Solid Edge part; units mm, degrees
sketch "Sketch1" plane through (0, 0, 2) normal (0, 0, 1) x (1, 0, 0)
  line L0 (49.4528, -16.8553) -> (36.691, -28.1957)
  arc A0 (31.6813, -30.1) -> (36.691, -28.1957) centre (35.1183, -31.6) cw
  line L1 (-5, -30.1) -> (31.6813, -30.1)
  line L2 (-5, -30.1) -> (-5, -33.1)
  line L3 (-5, -33.1) -> (31.6813, -33.1)
  line L4 (51.4456, -19.0978) -> (38.6838, -30.4383)
  arc A1 (38.6838, -30.4383) -> (31.6814, -33.1) centre (35.1183, -31.6) cw
  arc A2 (49.4528, -16.8553) -> (51.4456, -19.0978) centre (35.1183, -31.6) cw
  circle A3 centre (35.1183, -31.6) radius 1.75
extrude "ExtrudedProtrusion_1" add sketch "Sketch1" along normal blind 16.8
sketch "Sketch2" plane through (23.2228, -26.1027, 18.8) normal (0, 0, 1) x (-0.7475083, -0.6642525, 0)
  line L0 (-8.6773, 10.5109) -> (-25.7984, 3.6459)
  line L1 (-25.7984, 3.6459) -> (-25.7497, 10.5109)
  arc A0 (-25.7984, 11.5109) -> (-25.7497, 10.5109) centre (-5.2403, 12.0109) ccw
  line L2 (-25.7984, 11.5109) -> (-8.6773, 10.5109)
extrude "ExtrudedCutout_1" cut sketch "Sketch2" against normal blind 126.644
sketch "Sketch3" plane through (23.2228, -26.4602, 18.8) normal (0, 0, 1) x (-0.7475083, -0.6642525, 0)
  line L0 (-24.0241, 11.1261) -> (-27.0554, 10.1886)
  line L1 (-27.0554, 13.3363) -> (-27.0554, 10.1886)
  line L2 (-24.0241, 13.3363) -> (-27.0554, 13.3363)
  line L3 (-24.0241, 13.3363) -> (-24.0241, 11.1261)
extrude "ExtrudedCutout_2" cut sketch "Sketch3" against normal blind 19.824
sketch "Sketch4" plane through (22.489, -27.0845, 18.8) normal (0, 0, 1) x (-0.7475083, -0.6642525, 0)
  line L0 (-9.878, 10.2644) -> (-11.124, 7.7451)
  line L1 (-19.7514, 11.2253) -> (-9.878, 10.2644)
  arc A0 (-22.5172, 11.3271) -> (-19.7514, 11.2253) centre (-21.9785, -11.6575) cw
  line L2 (-22.5172, 11.3271) -> (-24.9872, 11.3468)
  line L3 (-24.9872, 11.1468) -> (-24.9872, 11.3468)
  line L4 (-24.9872, 11.1468) -> (-25.1125, 10.9171)
  line L5 (-25.1125, 10.9171) -> (-25.1125, 10.3529)
  arc A1 (-25.1125, 10.3529) -> (-11.1241, 7.7451) centre (-21.9785, -11.6575) cw
extrude "ExtrudedCutout_3" cut sketch "Sketch4" against normal blind 23.352
properties material "ABS Plastic, high impact"
For this review, take the finished solid that the model builds, in its own axes (mm). A direction names the side the tool comes from. Give positions to 0.01 mm unless a question says otherwise; leave off trailing zeros. Loops run counter-clockwise (first coordinate to the right, second up) from the corner with the lowest first, then second, coordinate; pieces in that order, holes last. Notation, with made-up numbers: M -26,55.25 L 24,55.25 A30 cw 24,77.25 Z; hole C 33.25,31.25 d3. An arc over 180 degrees is marked long. Answer as a JSON object with one key per item and string values. Group by question number.
Q1. Mouldability with a two-part tool opening along X and no side actions: class faces 1 (the flat face through (44.41, -25.35, 10.28)), 2 (the cylindrical face through (33.75, -28.11, 10.28)), 3 (the cylindrical face through (36.525, -35.076, 10.282)) as +X half, -X half, draft (parallel to the pull), parting line (faces both ways), or undercut.
Q2. Add section D-D on x = 39.5. Give the boundary of the cut face in (y, z).
Q3. Tool access review of faces 4 (the flat face through (13, -30.1, 10)), 5 (the flat face through (49.35, -19.695, 10.518)), 6 (the flat face through (13, -33.1, 10)): name each direction out of +Z, -Z, +X, -X, +Y, -Y from which nothing blocks a thin tool from reaching the whole face with its end or side.
Q4. For probe 1 along Y at (x, z) = (20, 5.75); probe 2 along X at (y, z) = (-32.5, 17.25); probe 3 along X at (y, z) = (-33, 13.5), list the stretches that pass through material, from the lowest coordinate up. Write a range as [from, to].
Q5. Insertion check: P1, Ø2, axis at y = -25.5, z = 13, coming from the +X side; P2, Ø6, axis at y = -33.5, z = 7, coming from the -X side; P3, Ø1.5, axis at y = -23.5, z = 15.5, coming from the -X side; P4, Ø8, axis at x = 15, z = 10, coming from the +Y side. Each pin has a flat end and moves straight along its axis. Give the tip position at first contact, or say it passes through.
Q6. Add section B-B on z = 6.25. Give the boundary of the cut face in (x, y), and give its area (3 significant figures).
Q7. Add section A-A on y = -31.6. Give the boundary of the cut face in (x, z).
Q8. Add section C-C on x = 9. Give the boundary of the cut face in (y, z), and give its area (3 significant figures).
Checked values:
{
 "1": {"face 1": "+X half", "face 2": "undercut", "face 3": "parting line"},
 "2": {"outline": "M -29.71,2 L -26.15,2 L -26.15,18.8 L -29.71,18.8 Z"},
 "3": {"face 4": "+Z, -Z, -X, +Y", "face 5": "+Z, -Z, +X, +Y", "face 6": "+Z, -Z, -X, -Y"},
 "4": {"probe 1": "[-33.1, -30.1]", "probe 2": "[-5, 33.62], [36.62, 38.76]", "probe 3": "[-5, 34.07], [36.17, 38.6]"},
 "5": {"P1": "x = 45.37", "P2": "x = -5", "P3": "x = 42.11", "P4": "y = -30.1"},
 "6": {"outline": "M -5,-33.1 L 31.68,-33.1 A3.75 ccw 38.68,-30.44 L 49.98,-20.4 L 48.7,-18.97 L 46.84,-20.59 A22.99 cw 44.71,-22.36 L 36.69,-28.2 A3.75 ccw 31.68,-30.1 L -5,-30.1 Z; hole C 35.12,-31.6 d3.5", "area": "178 mm²"},
 "7": {"outline": "M -5,2 L 33.37,2 L 33.37,18.8 L -5,18.8 Z; M 36.87,2 L 38.87,2 L 38.87,18.8 L 36.87,18.8 Z"},
 "8": {"outline": "M -33.1,2 L -30.1,2 L -30.1,18.8 L -33.1,18.8 Z", "area": "50.4 mm²"}
}
